```python
from build123d import *

# Parameters (mm, degrees)
SZKIC6_R                               = 4.5
WYTNIJ_WYCI_GNI_CIE1_DEPTH             = 6.5
WYTNIJ_WYCI_GNI_CIE2_REACH             = 5.5
SZKIC7_R                               = 2.5
WYTNIJ_WYCI_GNI_CIE2_DIRECTION_2_DEPTH = 7.5


with BuildPart() as part:
    # Szkic5 → Obrót1 (revolve)
    with BuildSketch(Plane(origin=(0, 0, 0), x_dir=(0, 0, -1), z_dir=(1, 0, 0))):
        Polygon((0, 10), (-9, 10), (-10, 0), (0, 0), align=None)
    revolve(axis=Axis((0, 0, 0), (0, 1, 0)))

    # Szkic6 → Wytnij-wyciągnięcie1 (cut)
    with BuildSketch(Plane(origin=(0, 10, 0), x_dir=(1, 0, 0), z_dir=(0, 1, 0))):
        Circle(SZKIC6_R)
    extrude(amount=-WYTNIJ_WYCI_GNI_CIE1_DEPTH, mode=Mode.SUBTRACT)

    # Szkic7 → Wytnij-wyciągnięcie2 (cut, up to next)
    with BuildSketch(Plane(origin=(0, 3.5, 0), x_dir=(1, 0, 0), z_dir=(0, 1, 0)), mode=Mode.PRIVATE) as wytnij_wyci_gni_cie2_sk1:
        Circle(SZKIC7_R)
    wytnij_wyci_gni_cie2_tool1 = extrude(wytnij_wyci_gni_cie2_sk1.sketch, amount=-WYTNIJ_WYCI_GNI_CIE2_REACH, mode=Mode.PRIVATE) & part.part
    add(wytnij_wyci_gni_cie2_tool1.solids().sort_by_distance((0, 3.5, 0))[0], mode=Mode.SUBTRACT)

    # Szkic7 → Wytnij-wyciągnięcie2 direction 2 (cut)
    with BuildSketch(Plane(origin=(0, 3.5, 0), x_dir=(1, 0, 0), z_dir=(0, 1, 0))):
        Circle(SZKIC7_R)
    extrude(amount=WYTNIJ_WYCI_GNI_CIE2_DIRECTION_2_DEPTH, mode=Mode.SUBTRACT)


solid = part.part
```
Could you check a few things on this model? Use its own coordinates, in mm. A direction names the side the tool comes from. Give positions to 0.01 mm unless a question says otherwise; leave off trailing zeros. Order: outer loops, then holes, each group sorted by start corner. A loop starts at its lowest first (then second) coordinate and runs counter-clockwise, first axis right, second up.
Q1. We'd pull the mould along Z, two halves only. Please class faces 3 (the flat face through (-2, 0, 2)), 4 (the conical face through (2.822, 6.041, 8.962)), 5 (the cylindrical face through (-0.54, 1.77, 2.44)): +Z half, -Z half, draft (parallel to the pull), parting line (faces both ways), or undercut.
Q2. Suppose I cut it at D-D, the plane y = 5. Write out the boundary of the cut face in (x, z), and give its area (3 significant figures).
Q3. For faces 1 (the flat face through (-4, 10, -4)), 2 (the flat face through (2, 3.5, 2)), which set-ups out of +Z, -Z, +X, -X, +Y, -Y let a thin tool reach every point of the face, with its end or its side?
Q4. Suppose I cut it at A-A, the plane z = 0. Write out the boundary of the cut face in (x, y), and give its area (3 significant figures).
Q5. Suppose I cut it at B-B, the plane x = 0. Write out the boundary of the cut face in (y, z).
Q6. Suppose I cut it at C-C, the plane y = 6.5. Write out the boundary of the cut face in (x, z), and give its area (3 significant figures).
Q7. If I drill on line 1 along Z through (x, y) = (0, 7.25) (3 decimals); line 2 along Y through (x, z) = (-0.75, 2.5); line 3 along X through (y, z) = (7, 3), over which ranges is the centre line in solid material (lowest first)?
Q8. I'm going to push flat-ended pins straight in: P1, Ø6, axis at y = 3, z = 5.5, coming from the -X side; P2, Ø1, axis at y = 3.5, z = 0, coming from the -X side; P3, Ø8, axis at x = 0, z = 0, coming from the +Y side. Where does each tip first touch, or does it pass through?
Solution:
1. face 3: draft
1. face 4: parting line
1. face 5: undercut
2. outline: circle Ø19 at (0, 0); hole circle Ø9 at (0, 0)
2. area: 220 mm2
3. face 1: +Z, -Z, +X, -X, +Y
3. face 2: +Y
4. outline: (-10, 0) - (-2.5, 0) - (-2.5, 3.5) - (-4.5, 3.5) - (-4.5, 10) - (-9, 10) - close; (2.5, 0) - (10, 0) - (9, 10) - (4.5, 10) - (4.5, 3.5) - (2.5, 3.5) - close
4. area: 114 mm2
5. outline: (0, -10) - (10, -9) - (10, -4.5) - (3.5, -4.5) - (3.5, -2.5) - (0, -2.5) - close; (0, 2.5) - (3.5, 2.5) - (3.5, 4.5) - (10, 4.5) - (10, 9) - (0, 10) - close
6. outline: circle Ø18.7 at (0, 0); hole circle Ø9 at (0, 0)
6. area: 211 mm2
7. line 1: z = -9.275 to -4.5, 4.5 to 9.275
7. line 2: y = 0 to 3.5
7. line 3: x = -8.8 to -3.35, 3.35 to 8.8
8. P1: stops at x = -9.43
8. P2: stops at x = -9.7
8. P3: stops at y = 3.5
